from build123d import *

# Parameters (mm, degrees)
F0_R           = 3.1
F0_W           = 53
F0_H           = 5
F0_R_2         = 2.1
F1_DEPTH       = 5
F2_DEPTH       = 2.1
F3_DEPTH       = 18
F4_W           = 0.8
F4_H           = 1
F4_W_2         = 51.4
F5_DEPTH       = 0.8
F6_DEPTH       = 25
F7_D           = 4
F7_CBORE_D     = 6.6
F7_CBORE_DEPTH = 3
F8_SIZE        = 2.5
F9_R           = 1.5
F10_SIZE       = 3


with BuildPart() as f1:
    # F0 (on Top) → F1 (new body)
    with BuildSketch(Plane.XY):
        with BuildLine():
            Line((26.5, -5), (-26.5, -5))
            Line((-26.5, -5), (-26.5, -27))
            Line((-26.5, -27), (1.616969722, -27))
            ThreePointArc((1.616969722, -27), (2.0486424192, -21.7348242496), (6.55, -24.5))
            ThreePointArc((6.55, -24.5), (6.2151757504, -25.9013575808), (5.283030278, -27))
            Line((5.283030278, -27), (26.5, -27))
            Line((26.5, -27), (26.5, -5))
        make_face()
        with Locations((-20.95, -9.5)):
            Circle(F0_R, mode=Mode.SUBTRACT)
        with Locations((20.95, -9.5)):
            Circle(F0_R, mode=Mode.SUBTRACT)
        with Locations((0, -2.5)):
            Rectangle(F0_W, F0_H)
        with Locations((-20.95, -9.5)):
            Circle(F0_R)
        with Locations((-20.95, -9.5)):
            Circle(F0_R_2, mode=Mode.SUBTRACT)
        with Locations((20.95, -9.5)):
            Circle(F0_R)
        with Locations((20.95, -9.5)):
            Circle(F0_R_2, mode=Mode.SUBTRACT)
    extrude(amount=F1_DEPTH)

    # F0 (on Top) → F2 (cut)
    with BuildSketch(Plane.XY):
        with Locations((20.95, -9.5)):
            Circle(F0_R)
        with Locations((20.95, -9.5)):
            Circle(F0_R_2, mode=Mode.SUBTRACT)
        with Locations((-20.95, -9.5)):
            Circle(F0_R)
        with Locations((-20.95, -9.5)):
            Circle(F0_R_2, mode=Mode.SUBTRACT)
    extrude(amount=F2_DEPTH, mode=Mode.SUBTRACT)

    # F0 (on Top) → F3 (join)
    with BuildSketch(Plane.XY):
        with Locations((0, -2.5)):
            Rectangle(F0_W, F0_H)
    extrude(amount=F3_DEPTH)

    # F4 (on face) → F5 (cut)
    with BuildSketch(Plane(origin=(0, 0, 0), x_dir=(-1, 0, 0), z_dir=(0, 1, 0))):
        with Locations((-26.1, 17.5)):
            Rectangle(F4_W, F4_H)
        with Locations((0, 17.5)):
            Rectangle(F4_W_2, F4_H)
        with Locations((26.1, 17.5)):
            Rectangle(F4_W, F4_H)
    extrude(amount=-F5_DEPTH, mode=Mode.SUBTRACT)

    # F4 (on face) → F6 (cut)
    with BuildSketch(Plane(origin=(0, 0, 0), x_dir=(-1, 0, 0), z_dir=(0, 1, 0))):
        with Locations((-26.1, 17.5)):
            Rectangle(F4_W, F4_H)
        with Locations((26.1, 17.5)):
            Rectangle(F4_W, F4_H)
    extrude(amount=-F6_DEPTH, mode=Mode.SUBTRACT)

    # F7 (through all)
    with Locations(Plane(origin=(0, 0, 0), x_dir=(-1, 0, 0), z_dir=(0, 1, 0))):
        with Locations((13.5, 10), (-13.5, 10)):
            CounterBoreHole(F7_D / 2, F7_CBORE_D / 2, F7_CBORE_DEPTH)

    # F8
    f8_edges = [f1.edges().sort_by_distance(p)[0] for p in [
        (0, -5, 18),
    ]]
    chamfer(f8_edges, length=F8_SIZE)

    # F9
    f9_edges = [f1.edges().sort_by_distance(p)[0] for p in [
        (0, -5, 5),
    ]]
    fillet(f9_edges, radius=F9_R)

    # F10
    f10_edges = [f1.edges().sort_by_distance(p)[0] for p in [
        (15.891515, -27, 5),
        (-12.441515, -27, 5),
    ]]
    chamfer(f10_edges, length=F10_SIZE)


solid = f1.part
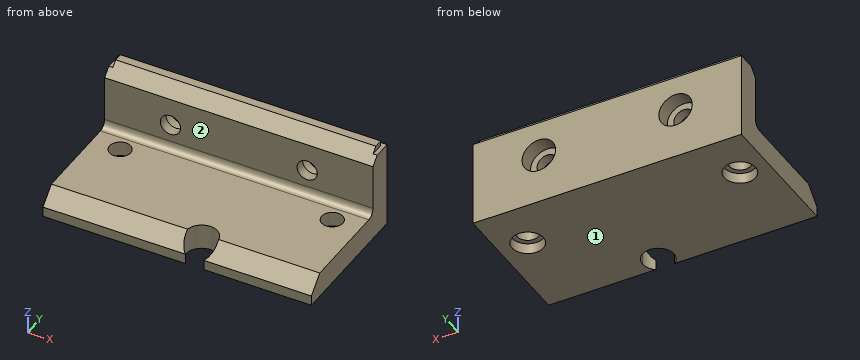
Verification items for the finished model (mm, model axes). Face numbers are marked on the shaded views. A direction names the side the tool comes from. Round coordinates to 2 decimals unless told otherwise and drop trailing zeros. Loops run counter-clockwise (first coordinate to the right, second up) from the corner with the lowest first, then second, coordinate; pieces in that order, holes last. Notation, with made-up numbers: (-21.75, 25) - (23.25, 25) arc R16 cw to (23.25, 30) - close; hole circle Ø5 at (3.5, -19). An arc over 180 degrees is marked (long way). Write item = value, one per line.
Q1. Sectioned sample at D-D on x = 3.45. Record the boundary of the cut face in (y, z).
Here are the results:
outline = (-21.4, 0) - (0, 0) - (0, 17) - (-0.8, 17) - (-0.8, 18) - (-2.5, 18) - (-5, 15.5) - (-5, 6.5) arc R1.5 cw to (-6.5, 5) - (-21.4, 5) - close
Q2. Sectioned sample at C-C on x = 20.95. Record the boundary of the cut face in (y, z), plus the area to 3 significant figures.
Here are the results:
outline = (-27, 0) - (-12.6, 0) - (-12.6, 2.1) - (-11.6, 2.1) - (-11.6, 5) - (-24, 5) - (-27, 2) - close; (-7.4, 2.1) - (-6.4, 2.1) - (-6.4, 0) - (0, 0) - (0, 17) - (-0.8, 17) - (-0.8, 18) - (-2.5, 18) - (-5, 15.5) - (-5, 6.5) arc R1.5 cw to (-6.5, 5) - (-7.4, 5) - close
area = 167 mm^2
Q3. Sectioned sample at B-B on z = 10. Record the boundary of the cut face in (x, y), plus the area to 3 significant figures.
Here are the results:
outline = (-26.5, -5) - (-15.5, -5) - (-15.5, -3) - (-16.8, -3) - (-16.8, 0) - (-26.5, 0) - close; (-11.5, -5) - (11.5, -5) - (11.5, -3) - (10.2, -3) - (10.2, 0) - (-10.2, 0) - (-10.2, -3) - (-11.5, -3) - close; (15.5, -5) - (26.5, -5) - (26.5, 0) - (16.8, 0) - (16.8, -3) - (15.5, -3) - close
area = 209 mm^2
Q4. Depth check by flat-ended pin: pin 1 (8 mm diameter, centred on x = -18, z = 6.5, fed in from +Y); pin 2 (2 mm diameter, centred on x = -13.5, z = 11.5, fed in from +Y); pin 3 (5 mm diameter, centred on x = 13.5, z = 10, fed in from -Y); pin 4 (10 mm diameter, centred on x = 20.95, y = -9.5, fed in from +Z). Enter the tip coordinate at first touch or a pass-through.
Here are the results:
pin_1 = 0
pin_2 = -3
pin_3 = -5
pin_4 = 16
Q5. Material ranges on L1, parallel to X at y = -4.25, z = 11.75; L2, parallel to Z at x = 13.5, y = -2.35; L3, parallel to Z at x = 13.5, y = -0.65, recorded low to high.
Here are the results:
L1 = -26.5 to -14.47, -12.53 to 12.53, 14.47 to 26.5
L2 = 0 to 6.7, 13.3 to 18
L3 = 0 to 6.7, 13.3 to 17
Q6. Tool access check on the marked faces 1 and 2. Record the directions out of +Z, -Z, +X, -X, +Y, -Y that give a thin tool (end or side, any length) a straight path to the whole face; none if there is none.
Here are the results:
face_1 = -Z, +X, -X, +Y, -Y
face_2 = +Z, +X, -X, -Y
Q7. Sectioned sample at A-A on y = -9.5. Record the boundary of the cut face in (x, z).
Here are the results:
outline = (-26.5, 0) - (-24.05, 0) - (-24.05, 2.1) - (-23.05, 2.1) - (-23.05, 5) - (-26.5, 5) - close; (-18.85, 2.1) - (-17.85, 2.1) - (-17.85, 0) - (17.85, 0) - (17.85, 2.1) - (18.85, 2.1) - (18.85, 5) - (-18.85, 5) - close; (23.05, 2.1) - (24.05, 2.1) - (24.05, 0) - (26.5, 0) - (26.5, 5) - (23.05, 5) - close
